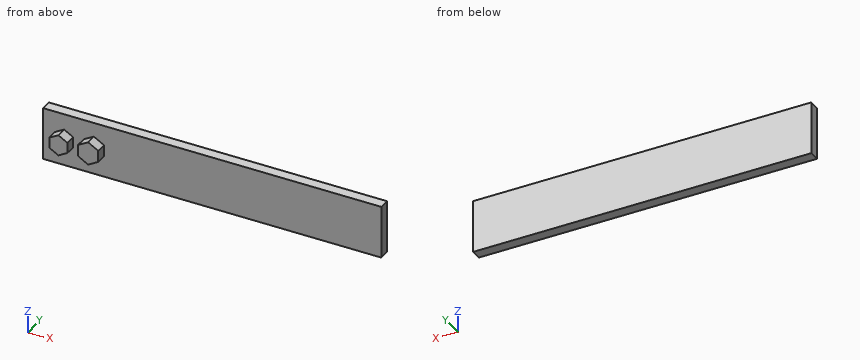
from build123d import *

# Parameters (mm, degrees)
F0_W     = 203.2
F0_H     = 31.75
F1_DEPTH = 6.35
F3_DEPTH = 6.35
F5_DEPTH = 6.35


with BuildPart() as f1:
    # F0 (on Front) → F1 (new body)
    with BuildSketch(Plane.XZ):
        with Locations((101.6, 15.875)):
            Rectangle(F0_W, F0_H)
    extrude(amount=F1_DEPTH)

    # F2 (on face) → F3 (join)
    with BuildSketch(Plane.XZ.offset(6.35)):
        Polygon((18.160766, 12.722225), (18.160766, 19.027775), (12.7, 22.18055), (7.239234, 19.027775), (7.239234, 12.722225), (12.7, 9.56945), align=None)
    extrude(amount=F3_DEPTH)

    # F4 (on face) → F5 (join)
    with BuildSketch(Plane.XZ.offset(6.35)):
        Polygon((36.609141, 12.722225), (36.609141, 19.707225), (30.559954, 23.199725), (24.510766, 19.707225), (24.510766, 12.722225), (30.559954, 9.229725), align=None)
    extrude(amount=F5_DEPTH)


solid = f1.part
Work out the finished part from the listing and answer in its coordinate system (mm). Give positions to 0.01 mm unless a question says otherwise; leave off trailing zeros. Loops run counter-clockwise (first coordinate to the right, second up) from the corner with the lowest first, then second, coordinate; pieces in that order, holes last. Notation, with made-up numbers: (45.25, -33.5) - (58.25, -33.5) arc R32 cw to (58.25, -4.5) - close; hole circle Ø4 at (72.25, 31). An arc over 180 degrees is marked (long way). Answer in a Markdown table with one row per item.
(1) Section C-C (x = 100) is taken. Give the vertices of the cut face in (y, z).
Results list:
| item | result |
|---|---|
| outline | (-6.35, 0) - (0, 0) - (0, 31.75) - (-6.35, 31.75) - close |
(2) Section B-B (z = 28.5) is taken. Give the vertices of the cut face in (x, y), and give its area (3 significant figures).
Results list:
| item | result |
|---|---|
| outline | (0, -6.35) - (203.2, -6.35) - (203.2, 0) - (0, 0) - close |
| area | 1,290 mm² |
(3) Consider L1, parallel to X at y = -11.25, z = 17; L2, parallel to Y at x = 112.5, z = 11; L3, parallel to X at y = -10.25, z = 12.5. Determine where each line is inside the solid, lowest interval first. Write a range as [from, to].
Results list:
| item | result |
|---|---|
| L1 | x = [7.24, 18.16], [24.51, 36.61] |
| L2 | y = [-6.35, 0] |
| L3 | x = [7.62, 17.78], [24.9, 36.22] |
(4) Flat-ended cylindrical pins translate along their axes: pin 1 Ø7 at (y, z) = (-11, 14.5) entering from +X; pin 2 Ø3 at (y, z) = (-10, 17) entering from -X. Find the tip coordinate at first contact, or state that the pin passes through.
Results list:
| item | result |
|---|---|
| pin 1 | stops at x = 36.61 |
| pin 2 | stops at x = 7.24 |
(5) Section A-A (y = -9) is taken. Give the vertices of the cut face in (x, z), and give its area (3 significant figures).
Results list:
| item | result |
|---|---|
| outline | (7.24, 12.72) - (12.7, 9.57) - (18.16, 12.72) - (18.16, 19.03) - (12.7, 22.18) - (7.24, 19.03) - close; (24.51, 12.72) - (30.56, 9.23) - (36.61, 12.72) - (36.61, 19.71) - (30.56, 23.2) - (24.51, 19.71) - close |
| area | 230 mm² |
